```python
from build123d import *

# Parameters (mm, degrees)
BOSS_EXTRUDE1_DEPTH         = 3.175
F_3_8_CLEARANCE_HOLE1_D     = 10.0838
F_3_8_CLEARANCE_HOLE1_DEPTH = 3.175
F_3_8_CLEARANCE_HOLE1_TIP   = 3.029479155


with BuildPart() as part:
    # Sketch1 → Boss-Extrude1 (new body)
    with BuildSketch(Plane(origin=(0, 0, 0), x_dir=(1, 0, 0), z_dir=(0, 1, 0))):
        Polygon((0, 0), (38.1, 0), (114.3, -76.2), (114.3, -114.3), (0, -114.3), align=None)
    extrude(amount=BOSS_EXTRUDE1_DEPTH)

    # 3/8 Clearance Hole1
    with Locations(Plane(origin=(0, 3.175, 0), x_dir=(1, 0, 0), z_dir=(0, 1, 0))):
        with Locations((19.05, -19.05), (19.05, -38.1), (19.05, -57.15), (19.05, -76.2), (38.1, -95.25), (57.15, -95.25), (76.2, -95.25), (95.25, -95.25)):
            Hole(F_3_8_CLEARANCE_HOLE1_D / 2, depth=F_3_8_CLEARANCE_HOLE1_DEPTH)
            with Locations((0, 0, -(F_3_8_CLEARANCE_HOLE1_DEPTH + F_3_8_CLEARANCE_HOLE1_TIP / 2))):  # 118° drill point
                Cone(0, F_3_8_CLEARANCE_HOLE1_D / 2, F_3_8_CLEARANCE_HOLE1_TIP, mode=Mode.SUBTRACT)


solid = part.part
```
Input: part model. Units: mm. Frame: model coordinates. Give positions to 0.01 mm unless a question says otherwise; leave off trailing zeros. Loops run counter-clockwise (first coordinate to the right, second up) from the corner with the lowest first, then second, coordinate; pieces in that order, holes last. Notation, with made-up numbers: (68, -21) -> (88, -21) arc R23 cw to (88, -11) -> close; hole circle Ø9 at (15.5, -39). An arc over 180 degrees is marked (long way). Use a Markdown table: item, result.
Q1. Section query B-B, the plane y = 2. State how many separate pieces and enclosed holes the cut face has, plus the area to 3 significant figures.
Entries:
| item | result |
|---|---|
| separate pieces | 1 |
| enclosed holes | 8 |
| area | 9,520 mm² |
Q2. Ray query, probe 1 along Z at (x, y) = (19, 2); probe 2 along X at (y, z) = (0.85, 95.25); probe 3 along X at (y, z) = (2.2, 38.1). Return the intervals inside material, ascending. Write a range as from..to.
Entries:
| item | result |
|---|---|
| probe 1 | z = 0..14.01, 24.09..33.06, 43.14..52.11, 62.19..71.16, 81.24..114.3 |
| probe 2 | x = 0..33.06, 43.14..52.11, 62.19..71.16, 81.24..90.21, 100.29..114.3 |
| probe 3 | x = 0..14.01, 24.09..76.2 |
Q3. Section query C-C, the plane z = 16. Return the cut outline in (x, y) (3 decimals).
Entries:
| item | result |
|---|---|
| outline | (0, 0) -> (15.035, 0) -> (15.035, 3.175) -> (0, 3.175) -> close; (23.065, 0) -> (54.1, 0) -> (54.1, 3.175) -> (23.065, 3.175) -> close |
Q4. Section query D-D, the plane x = 19.05. Return the cut outline in (y, z) (3 decimals), plus the area to 3 significant figures.
Entries:
| item | result |
|---|---|
| outline | (0, 0) -> (3.175, 0) -> (3.175, 14.008) -> (0, 14.008) -> close; (0, 24.092) -> (3.175, 24.092) -> (3.175, 33.058) -> (0, 33.058) -> close; (0, 43.142) -> (3.175, 43.142) -> (3.175, 52.108) -> (0, 52.108) -> close; (0, 62.192) -> (3.175, 62.192) -> (3.175, 71.158) -> (0, 71.158) -> close; (0, 81.242) -> (3.175, 81.242) -> (3.175, 114.3) -> (0, 114.3) -> close |
| area | 235 mm² |
Q5. Section query A-A, the plane x = 76.2. Return the cut outline in (y, z) (3 decimals).
Entries:
| item | result |
|---|---|
| outline | (0, 38.1) -> (3.175, 38.1) -> (3.175, 90.208) -> (0, 90.208) -> close; (0, 100.292) -> (3.175, 100.292) -> (3.175, 114.3) -> (0, 114.3) -> close |
Q6. Pull-direction query (Y, two-part tool) for faces 1 (the flat face through (45, 3.175, 69)), 2 (the cylindrical face through (20.143, 1.565, 43.022)), 3 (the flat face through (45, 0, 69)); classes: pulls with the +Y half, pulls with the -Y half, needs draft (parallel to the pull), parting line crosses it, or undercut.
Entries:
| item | result |
|---|---|
| face 1 | pulls with the +Y half |
| face 2 | needs draft |
| face 3 | pulls with the -Y half |
Q7. First-contact query: P1, Ø1.5, axis at y = 1.5, z = 42.5, coming from the +X side; P2, Ø9, axis at x = 19.05, z = 57.15, coming from the -Y side. Flat tips, straight axial feed; report the tip coordinate or a pass-through.
Entries:
| item | result |
|---|---|
| P1 | stops at x = 81.35 |
| P2 | passes through |
